Check sheet for the modelled part. Datum: model origin and axes. Units: mm. Face numbers are marked on the shaded views. A direction names the side the tool comes from. Round coordinates to 2 decimals unless told otherwise and drop trailing zeros. Order: outer loops, then holes, each group sorted by start corner. A loop starts at its lowest first (then second) coordinate and runs counter-clockwise, first axis right, second up. Notation, with made-up numbers: (39.25, -8) -> (58.25, -8) arc R15 ccw to (58.25, 12) -> close; hole circle Ø6 at (-37.75, -15.75). An arc over 180 degrees is marked (long way). Answer in a Markdown table with one row per item.
```python
from build123d import *

# Parameters (mm, degrees)
F2_DEPTH          = 3
F6_DEPTH          = 1.5
F9_DEPTH          = 26.2
F9_DEPTH_BACK     = 25
F10_R             = 1.5
F11_DEPTH         = 32.4
F13_R             = 2.25
F14_DEPTH         = 2
F14_COPIES2_COUNT = 2
F14_COPIES2_PITCH = 61.077819
F15_W             = 29
F15_H             = 11
F16_DEPTH         = 0.75


# Not quite as in the source:
# - a pattern or mirror of a feature is missing from the dataset's text; its kind, count and spacing are read off the source's solid


with BuildPart() as f2:
    # F1 (on offset) → F2 (new body)
    with BuildSketch(Plane.XY.offset(3.5)):
        Polygon((-25.25, -15.25), (-25.25, -2.5), (-25.25, 2.5), (-25.25, 15.25), (-30.25, 15.25), (-30.25, 0), (-30.25, -15.25), align=None)
        Polygon((0, -2.5), (25.25, -2.5), (25.25, 2.5), (0, 2.5), (-25.25, 2.5), (-25.25, -2.5), align=None)
        Polygon((30.25, -15.25), (30.25, 0), (30.25, 15.25), (25.25, 15.25), (25.25, 2.5), (25.25, -2.5), (25.25, -15.25), align=None)
    extrude(amount=F2_DEPTH)

    # F5 (on plane+point) → F6 (join, symmetric)
    with BuildSketch(Plane.YZ.offset(27.75)):
        Polygon((10.057664814, 6.5), (13.25, 6.5), (1.5, 38.8), (0, 38.8), (-1.5, 38.8), (-13.25, 6.5), (-10.057664814, 6.5), (-1.5, 30.0244743399), (0, 30.0244743399), (1.5, 30.0244743399), align=None)
    f6 = extrude(amount=F6_DEPTH, both=True)

    # F6_copies: F6 across plane
    add(f6.mirror(Plane(origin=(0, 0, 0), x_dir=(0, 0, -1), z_dir=(-1, 0, 0))))

    # F8 (on face) → F9 (join, two sides)
    with BuildSketch(Plane.XY.offset(38.8)) as f9_sk:
        with BuildLine():
            ThreePointArc((27.75, -1.5), (28.8106601718, -1.0606601718), (29.25, 0))
            ThreePointArc((29.25, 0), (28.8106601718, 1.0606601718), (27.75, 1.5))
            ThreePointArc((27.75, 1.5), (26.68933982, 1.0606601636), (26.25, -2.31e-08))
            ThreePointArc((26.25, -2.31e-08), (26.6893398364, -1.06066018), (27.75, -1.5))
        make_face()
    f9 = extrude(amount=F9_DEPTH) + extrude(f9_sk.sketch, amount=-F9_DEPTH_BACK)

    # F9_copies: F9 across plane
    add(f9.mirror(Plane(origin=(0, 0, 0), x_dir=(0, 0, -1), z_dir=(-1, 0, 0))))

    # F10 (on Right) → F11 (join, symmetric)
    with BuildSketch(Plane.YZ):
        with Locations((0, 65)):
            Circle(F10_R)
    extrude(amount=F11_DEPTH, both=True)

    # F13 (on offset) → F14 (join)
    with BuildSketch(Plane.XZ.offset(13.75)):
        with Locations((27.75, 2.25)):
            Circle(F13_R)
    f14 = extrude(amount=-F14_DEPTH)

    # F14_copies: F14 across plane
    add(f14.mirror(Plane.ZX))

    # F14_copies1: F14 across plane
    add(f14.mirror(Plane(origin=(0, 0, 0), x_dir=(0, 0, -1), z_dir=(-1, 0, 0))))

    # F14_copies2: F14 ×2
    with Locations(*[Vector(-0.908676844, 0.4175001716, 0) * (i * F14_COPIES2_PITCH) for i in range(1, F14_COPIES2_COUNT)]):
        add(f14)

    # F15 (on Front) → F16 (join, symmetric)
    with BuildSketch(Plane.XZ):
        with Locations((0, 71.5)):
            Rectangle(F15_W, F15_H)
    extrude(amount=F16_DEPTH, both=True)


solid = f2.part
```
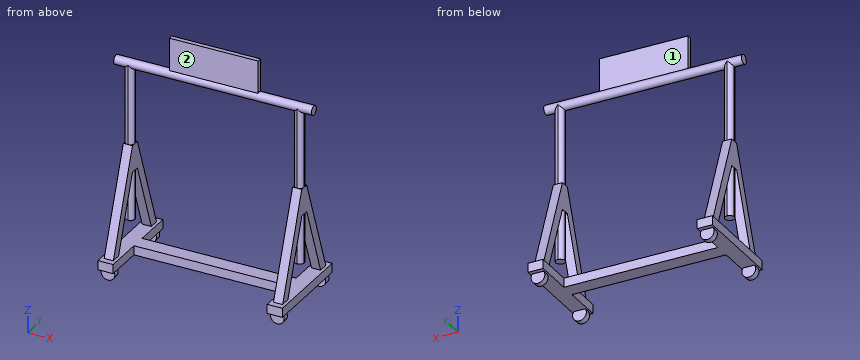
(1) Scan lines: probe 1 along X at (y, z) = (3, 28.5); probe 2 along X at (y, z) = (4, 4); probe 3 along Z at (x, y) = (4, -0.5). Record each from-to range of solid material in increasing order. Write a range as from..to.
Solutions:
| item | result |
|---|---|
| probe 1 | -29.25..-26.25, 26.25..29.25 |
| probe 2 | -30.25..-25.25, 25.25..30.25 |
| probe 3 | 3.5..6.5, 63.59..77 |
(2) Depth check by flat-ended pin: pin 1 Ø1.7 at (y, z) = (0.5, 69) entering from +X; pin 2 Ø2.5 at (y, z) = (-9.5, 4.5) entering from -X; pin 3 Ø1 at (x, z) = (28, 2.5) entering from -Y; pin 4 Ø12 at (x, y) = (-5.5, -9) entering from +Z. Enter the tip coordinate at first touch or a pass-through.
Solutions:
| item | result |
|---|---|
| pin 1 | x = 14.5 |
| pin 2 | x = -30.25 |
| pin 3 | y = -13.75 |
| pin 4 | through |
(3) Section check B-B on z = 45.5. Record the boundary of the cut face in (x, y), plus the area to 3 significant figures.
Solutions:
| item | result |
|---|---|
| outline | circle Ø3 at (-27.75, 0); circle Ø3 at (27.75, 0) |
| area | 14.1 mm^2 |
(4) Section check D-D on y = 3.5. Record the boundary of the cut face in (x, z).
Solutions:
| item | result |
|---|---|
| outline | (-30.25, 3.5) -> (-25.25, 3.5) -> (-25.25, 6.5) -> (-30.25, 6.5) -> close; (-29.25, 24.53) -> (-26.25, 24.53) -> (-26.25, 33.3) -> (-29.25, 33.3) -> close; (25.25, 3.5) -> (30.25, 3.5) -> (30.25, 6.5) -> (25.25, 6.5) -> close; (26.25, 24.53) -> (29.25, 24.53) -> (29.25, 33.3) -> (26.25, 33.3) -> close |
(5) Tool access check on the marked faces 1 and 2. Record the directions out of +Z, -Z, +X, -X, +Y, -Y that give a thin tool (end or side, any length) a straight path to the whole face; none if there is none.
Solutions:
| item | result |
|---|---|
| face 1 | +Z, +X, -X, +Y |
| face 2 | +Z, +X, -X, -Y |
(6) Section check A-A on x = 16. Record the boundary of the cut face in (y, z).
Solutions:
| item | result |
|---|---|
| outline | (-2.5, 3.5) -> (2.5, 3.5) -> (2.5, 6.5) -> (-2.5, 6.5) -> close; circle Ø3 at (0, 65) |
(7) Section check C-C on z = 2.25. Record the boundary of the cut face in (x, y).
Solutions:
| item | result |
|---|---|
| outline | (-30, -13.75) -> (-25.5, -13.75) -> (-25.5, -11.75) -> (-30, -11.75) -> close; (-30, 11.75) -> (-25.5, 11.75) -> (-25.5, 13.75) -> (-30, 13.75) -> close; (25.5, -13.75) -> (30, -13.75) -> (30, -11.75) -> (25.5, -11.75) -> close; (25.5, 11.75) -> (30, 11.75) -> (30, 13.75) -> (25.5, 13.75) -> close |
